Verification items for the finished model (mm, model axes). Face numbers are marked on the shaded views. A direction names the side the tool comes from. Round coordinates to 2 decimals unless told otherwise and drop trailing zeros. Order: outer loops, then holes, each group sorted by start corner. A loop starts at its lowest first (then second) coordinate and runs counter-clockwise, first axis right, second up. Notation, with made-up numbers: (27.5, -37.75) -> (71.5, -37.75) arc R24 ccw to (71.5, -6.75) -> close; hole circle Ø8 at (32.25, 75.5). An arc over 180 degrees is marked (long way). Return JSON: item names as keys, results as strings. Group by question number.
Item 1: Depth check by flat-ended pin: pin 1 Ø8.5 at (x, y) = (-17.375, -34.5) entering from +Z; pin 2 Ø4 at (x, y) = (0, -45) entering from +Z; pin 3 Ø1.5 at (x, z) = (-21, 6) entering from -Y; pin 4 Ø2.5 at (x, y) = (-24.75, 45) entering from -Z. Enter the tip coordinate at first touch or a pass-through.
Item 2: Sectioned sample at C-C on z = 29. Record the cut outline in (x, y).
Item 3: Scan lines: probe 1 along Y at (x, z) = (-17, 17); probe 2 along X at (y, z) = (45, 0.6); probe 3 along Y at (x, z) = (0, 1). Record each from-to range of solid material in increasing order. Write a range as from..to.
Item 4: Sectioned sample at B-B on y = 45. Record the cut outline in (x, z), plus the area to 3 significant figures.
Item 5: Access from +Z, -Z, +X, -X, +Y, -Y to the whole of each face (thin tool, end or side, straight path). Record for the marked faces 1, 2, 3 and 4.
Item 6: Sectioned sample at A-A on x = -24.75. Record the cut outline in (y, z), plus the area to 3 significant figures.
Item 7: Sectioned sample at D-D on x = -9. Record the cut outline in (y, z), plus the area to 3 significant figures.
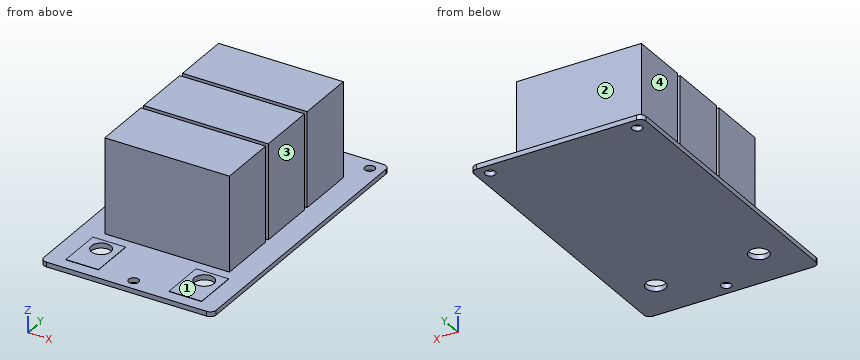
Autodesk Inventor part; units mm, degrees
ref_plane "YZ Plane" through (0, 0, 0) normal (1, 0, 0) x (0, 1, 0)
ref_plane "XZ Plane" through (0, 0, 0) normal (0, 1, 0) x (-1, 0, 0)
ref_plane "XY Plane" through (0, 0, 0) normal (0, 0, 1) x (1, 0, 0)
sketch "Sketch1" plane through (0, 0, 0) normal (0, 0, 1) x (1, 0, 0)
  line L0 (-29, -49) -> (29, -49)
  line L1 (29, -49) -> (29, 49)
  line L2 (29, 49) -> (-29, 49)
  line L3 (-29, 49) -> (-29, -49)
  line L4 (-29, -49) -> (29, 49) construction
  line L5 (29, -49) -> (-29, 49) construction
  point P0 (0, 0)
  dimension "d0" = 58
  dimension "d1" = 98
extrude "Extrusion1" add sketch "Sketch1" along normal blind 1.6
sketch "Sketch2" plane through (0, 0, 1.6) normal (0, 0, 1) x (1, 0, 0)
  line L0 (-21, 16.5) -> (21, 16.5)
  line L1 (21, 16.5) -> (21, 36.5)
  line L2 (21, 36.5) -> (-21, 36.5)
  line L3 (-21, 36.5) -> (-21, 16.5)
  line L4 (-21, 16.5) -> (21, 36.5) construction
  line L5 (21, 16.5) -> (-21, 36.5) construction
  line L6 (-21, -5) -> (21, -5)
  line L7 (21, -5) -> (21, 15)
  line L8 (21, 15) -> (-21, 15)
  line L9 (-21, 15) -> (-21, -5)
  line L10 (-21, -5) -> (21, 15) construction
  line L11 (21, -5) -> (-21, 15) construction
  line L12 (-21, -26.5) -> (21, -26.5)
  line L13 (21, -26.5) -> (21, -6.5)
  line L14 (21, -6.5) -> (-21, -6.5)
  line L15 (-21, -6.5) -> (-21, -26.5)
  line L16 (-21, -26.5) -> (21, -6.5) construction
  line L17 (21, -26.5) -> (-21, -6.5) construction
  line L18 (-29, -49) -> (29, -49)
  line L19 (29, 49) -> (-29, 49)
  point P0 (0, 0)
  point P1 (0, 26.5)
  point P2 (0, 5)
  point P3 (0, -16.5)
  point P4 (0, 16.5)
  dimension "d4" = 42
  dimension "d5" = 20
  dimension "d6" = 20
  dimension "d7" = 20
  dimension "d8" = 1.5
  dimension "d9" = 1.5
  dimension "d31" = 12.5
extrude "Extrusion2" add sketch "Sketch2" along normal blind 32
sketch "Sketch3" plane through (0, 0, 1.6) normal (0, 0, 1) x (1, 0, 0)
  line L0 (-24.75, -45) -> (24.75, -45) construction
  line L1 (24.75, -45) -> (24.75, 45) construction
  line L2 (24.75, 45) -> (-24.75, 45) construction
  line L3 (-24.75, 45) -> (-24.75, -45) construction
  line L4 (-24.75, -45) -> (24.75, 45) construction
  line L5 (24.75, -45) -> (-24.75, 45) construction
  point P0 (0, 0)
  point P1 (0, -45)
  dimension "d13" = 90
  dimension "d14" = 49.5
hole "Hole1" at (-24.75, 45, 1.6) at (24.75, 45, 1.6) at (0, -45, 1.6) direction (0, 0, -1) diameter 3.4 depth 9.525 tip angle 118
fillet "Fillet1" radius 2 4 edges at (29, 49, 0.8) (-29, 49, 0.8) (29, -49, 0.8) (-29, -49, 0.8)
sketch "Sketch4" plane through (0, 0, 1.6) normal (0, 0, 1) x (1, 0, 0)
  line L0 (-17.375, -34.5) -> (17.375, -34.5) construction
  circle A0 centre (24.75, -45) radius 1.7 construction
  line L1 (-27, -49) -> (27, -49)
  point P0 (0, 0)
  point P1 (0, -34.5)
  dimension "d23" = 34.75
  dimension "d32" = 14.5
hole "Hole2" at (-17.375, -34.5, 1.6) at (17.375, -34.5, 1.6) direction (0, 0, -1) diameter 6.6 depth 9.525 tip angle 118
sketch "Sketch5" plane through (0, 0, 1.6) normal (0, 0, 1) x (1, 0, 0)
  point P0 (0, 0)
sketch "Sketch6" plane through (0, 0, 1.6) normal (0, 0, 1) x (1, 0, 0)
  line L0 (-22.875, -45) -> (-11.875, -45)
  line L1 (-11.875, -45) -> (-11.875, -30)
  line L2 (-11.875, -30) -> (-22.875, -30)
  line L3 (-22.875, -30) -> (-22.875, -45)
  line L4 (-22.875, -45) -> (-11.875, -30) construction
  line L5 (-11.875, -45) -> (-22.875, -30) construction
  line L6 (11.875, -45) -> (22.875, -45)
  line L7 (22.875, -45) -> (22.875, -30)
  line L8 (22.875, -30) -> (11.875, -30)
  line L9 (11.875, -30) -> (11.875, -45)
  line L10 (11.875, -45) -> (22.875, -30) construction
  line L11 (22.875, -45) -> (11.875, -30) construction
  circle A0 centre (-17.375, -34.5) radius 3.3
  circle A1 centre (17.375, -34.5) radius 3.3
  point P0 (0, 0)
  point P1 (-17.375, -37.5)
  point P2 (17.375, -37.5)
  point P3 (-17.375, -37.5)
  point P4 (17.375, -37.5)
  dimension "d33" = 3
  dimension "d34" = 11
  dimension "d35" = 11
  dimension "d36" = 15
extrude "Extrusion3" add sketch "Sketch6" along normal blind 0.1
properties part number "Cap_Platine"
Recorded:
{
 "1": {"pin 1": "z = 1.7", "pin 2": "z = 1.6", "pin 3": "y = -26.5", "pin 4": "through"},
 "2": {"outline": "(-21, -26.5) -> (21, -26.5) -> (21, -6.5) -> (-21, -6.5) -> close; (-21, -5) -> (21, -5) -> (21, 15) -> (-21, 15) -> close; (-21, 16.5) -> (21, 16.5) -> (21, 36.5) -> (-21, 36.5) -> close"},
 "3": {"probe 1": "-26.5..-6.5, -5..15, 16.5..36.5", "probe 2": "-29..-26.45, -23.05..23.05, 26.45..29", "probe 3": "-49..-46.7, -43.3..49"},
 "4": {"outline": "(-29, 0) -> (-26.45, 0) -> (-26.45, 1.6) -> (-29, 1.6) -> close; (-23.05, 0) -> (23.05, 0) -> (23.05, 1.6) -> (-23.05, 1.6) -> close; (26.45, 0) -> (29, 0) -> (29, 1.6) -> (26.45, 1.6) -> close", "area": "81.9 mm²"},
 "5": {"face 1": "+Z, +X, -X, -Y", "face 2": "+Z, +X, -X, +Y", "face 3": "+Z, +X, +Y, -Y", "face 4": "+Z, -X, +Y, -Y"},
 "6": {"outline": "(-49, 0) -> (43.3, 0) -> (43.3, 1.6) -> (-49, 1.6) -> close; (46.7, 0) -> (49, 0) -> (49, 1.6) -> (46.7, 1.6) -> close", "area": "151 mm²"},
 "7": {"outline": "(-49, 0) -> (49, 0) -> (49, 1.6) -> (36.5, 1.6) -> (36.5, 33.6) -> (16.5, 33.6) -> (16.5, 1.6) -> (15, 1.6) -> (15, 33.6) -> (-5, 33.6) -> (-5, 1.6) -> (-6.5, 1.6) -> (-6.5, 33.6) -> (-26.5, 33.6) -> (-26.5, 1.6) -> (-49, 1.6) -> close", "area": "2,080 mm²"}
}
